```python
from build123d import *

# Parameters (mm, degrees)
SKETCH_W     = 12
SKETCH_H     = 16
PAD_DEPTH    = 3
CHAMFER_SIZE = 1
FILLET_R     = 1


with BuildPart() as part:
    # Sketch → Pad (new body)
    with BuildSketch(Plane.XY):
        with Locations((6, 8)):
            Rectangle(SKETCH_W, SKETCH_H)
        with BuildLine():
            ThreePointArc((4.25, 13), (3, 14.25), (1.75, 13))
            Line((1.75, 13), (1.75, 3))
            ThreePointArc((1.75, 3), (3, 1.75), (4.25, 3))
            Line((4.25, 13), (4.25, 3))
        make_face(mode=Mode.SUBTRACT)
        with BuildLine():
            ThreePointArc((10.25, 13), (9, 14.25), (7.75, 13))
            Line((7.75, 13), (7.75, 3))
            ThreePointArc((7.75, 3), (9, 1.75), (10.25, 3))
            Line((10.25, 13), (10.25, 3))
        make_face(mode=Mode.SUBTRACT)
    extrude(amount=PAD_DEPTH)

    # Chamfer
    chamfer_edges = [part.edges().sort_by_distance(p)[0] for p in [
        (4.25, 8, 3),
        (4.25, 8, 0),
        (10.25, 8, 0),
        (10.25, 8, 3),
    ]]
    chamfer(chamfer_edges, length=CHAMFER_SIZE)

    # Fillet
    fillet_edges = [part.edges().sort_by_distance(p)[0] for p in [
        (0, 16, 1.5),
        (0, 0, 1.5),
        (12, 0, 1.5),
        (12, 16, 1.5),
    ]]
    fillet(fillet_edges, radius=FILLET_R)


solid = part.part
```
Check sheet for the modelled part. Datum: model origin and axes. Units: mm. A direction names the side the tool comes from. Give positions to 0.01 mm unless a question says otherwise; leave off trailing zeros. Order: outer loops, then holes, each group sorted by start corner. A loop starts at its lowest first (then second) coordinate and runs counter-clockwise, first axis right, second up. Notation, with made-up numbers: M 49,-21.5 L 89,-21.5 A29 cw 89,6.5 Z; hole C 56.5,59 d9. An arc over 180 degrees is marked long. Answer in a Markdown table with one row per item. Add a question column.
Q1. Gauge pin test, flat end, axial feed: pin 1 Ø2 at (x, y) = (9, 13.5) entering from -Z. Record the tip position at first contact, or that the pin passes through.
Q2. Release check for a two-part mould opening along X. For faces 5 (the flat face through (1.24, 7.93, 0.49)), 6 (the cylindrical face through (11.699, 15.715, 1.521)), 7 (the cylindrical face through (3.03, 14.25, 1.49)), 8 (the cylindrical face through (0.285, 15.699, 1.521)) record: released by +X, released by -X, zero draft, split by the parting line, or undercut.
Q3. Sectioned sample at C-C, the plane y = 9.5. Record the boundary of the cut face in (x, z).
Q4. Sectioned sample at A-A, the plane x = 9. Record the boundary of the cut face in (y, z).
Q5. Thickness scan on L1, parallel to X at y = 11.75, z = 1.75; L2, parallel to X at y = 6.75, z = 0.4; L3, parallel to Y at x = 10.5, z = 0.2. Record the ranges inside material, lowest first.
Q6. Access from +Z, -Z, +X, -X, +Y, -Y to the whole of each face (thin tool, end or side, straight path). Record for faces 1 (the flat face through (6, 0, 1)), 2 (the flat face through (10.25, 8.1, 1.5)), 3 (the flat face through (1.24, 7.93, 2.51)), 4 (the conical face through (9.03, 1.58, 0.83)).
Q7. Sectioned sample at D-D, the plane z = 1.8. Record the boundary of the cut face in (x, y), and give its area (3 significant figures).
Q8. Sectioned sample at B-B, the plane z = 0.2. Record the boundary of the cut face in (x, y), and give its area (3 significant figures).
Verdict:
| question | item | result |
|---|---|---|
| 1 | pin 1 | z = 0.75 |
| 2 | face 5 | undercut |
| 2 | face 6 | released by +X |
| 2 | face 7 | undercut |
| 2 | face 8 | released by -X |
| 3 | outline | M 0,0 L 0.75,0 L 1.75,1 L 1.75,2 L 0.75,3 L 0,3 Z; M 4.25,1 L 5.25,0 L 6.75,0 L 7.75,1 L 7.75,2 L 6.75,3 L 5.25,3 L 4.25,2 Z; M 10.25,1 L 11.25,0 L 12,0 L 12,3 L 11.25,3 L 10.25,2 Z |
| 4 | outline | M 0,0 L 0.75,0 L 1.75,1 L 1.75,2 L 0.75,3 L 0,3 Z; M 14.25,1 L 15.25,0 L 16,0 L 16,3 L 15.25,3 L 14.25,2 Z |
| 5 | L1 | 0 to 1.75, 4.25 to 7.75, 10.25 to 12 |
| 5 | L2 | 0 to 1.15, 4.85 to 7.15, 10.85 to 12 |
| 5 | L3 | 0 to 1.6, 14.4 to 16 |
| 6 | face 1 | +Z, -Z, +X, -X, -Y |
| 6 | face 2 | +Z, -Z |
| 6 | face 3 | +Z |
| 6 | face 4 | -Z |
| 7 | outline | M 0,1 A1 ccw 1,0 L 11,0 A1 ccw 12,1 L 12,15 A1 ccw 11,16 L 1,16 A1 ccw 0,15 Z; hole M 1.75,3 A1.25 ccw 4.25,3 L 4.25,13 A1.25 ccw 1.75,13 Z; hole M 7.75,3 A1.25 ccw 10.25,3 L 10.25,13 A1.25 ccw 7.75,13 Z |
| 7 | area | 131 mm² |
| 8 | outline | M 0,1 A1 ccw 1,0 L 11,0 A1 ccw 12,1 L 12,15 A1 ccw 11,16 L 1,16 A1 ccw 0,15 Z; hole M 0.95,3 A2.05 ccw 5.05,3 L 5.05,13 A2.05 ccw 0.95,13 Z; hole M 6.95,3 A2.05 ccw 11.05,3 L 11.05,13 A2.05 ccw 6.95,13 Z |
| 8 | area | 82.7 mm² |
